```python
from build123d import *
from build123d import SkipClean  # not in build123d's __all__

# Parameters (mm, degrees)
F0_W             = 57.5
F0_H             = 50
F1_DEPTH         = 107.5
F2_W             = 55.8
F2_H             = 19
F3_DEPTH         = 42
F4_W             = 0.3
F4_H             = 19
F5_DEPTH         = 48.3
F6_T1_DEPTH      = 65.5
F6_T3_DEPTH      = 67.5
F6_T5_DEPTH      = 225
F6_T7_DEPTH      = 11.7
F6_T9_DEPTH      = 11.7
F6_T11_DEPTH     = 204
F8_W             = 87
F8_H             = 15.3
F9_DEPTH         = 14
F10_W            = 8.2
F10_H            = 14
F11_DEPTH        = 7.4
F12_R            = 2
F13_R            = 2.5
F14_DEPTH        = 4
F15_R            = 1
F19_D            = 3.3
F19_DEPTH        = 5
F19_TIP          = 0.9914200214
F19_ON_F18_D     = 3.3
F19_ON_F18_DEPTH = 5
F19_ON_F18_TIP   = 0.9914200214
F19_ON_F17_D     = 3.3
F19_ON_F17_DEPTH = 5
F19_ON_F17_TIP   = 0.9914200214
F20_W            = 264
F20_H            = 50
F20_R            = 1.5
F21_DEPTH        = 6
F22_W            = 122
F22_H            = 91
F22_R            = 2.25
F23_DEPTH        = 2.4
F24_W            = 91
F24_H            = 52.9
F24_R            = 1.75
F25_DEPTH        = 2.4
F26_R            = 2.25
F27_DEPTH        = 25
F28_W            = 91
F28_H            = 52.9
F29_DEPTH        = 3
F30_R            = 1.75
F31_DEPTH        = 25
F32_W            = 127.4
F32_H            = 91
F33_DEPTH        = 2.4
F34_W            = 127.4
F34_H            = 55.3
F34_R            = 6.5
F35_DEPTH        = 2.4
F36_W            = 21.5
F36_H            = 28.5
F37_DEPTH        = 25
F38_W            = 20
F38_H            = 100
F39_DEPTH        = 60
F43_W            = 2.4
F43_H            = 50.5
F44_DEPTH        = 45


# Not quite as in the source:
# - a fillet or chamfer that OpenCascade refuses, or shapes differently, is made with other operations: its cross-section is extruded or revolved along the edge and cut away or added


with BuildPart() as f1:
    # F0 (on Front) → F1 (new body, symmetric)
    with BuildSketch(Plane.XZ):
        with Locations((-28.75, 0)):
            Rectangle(F0_W, F0_H)
    extrude(amount=F1_DEPTH, both=True)

    # F2 (on face) → F3 (cut)
    with BuildSketch(Plane.XY.offset(25)):
        with Locations((-27.9, -98)):
            Rectangle(F2_W, F2_H)
    extrude(amount=-F3_DEPTH, mode=Mode.SUBTRACT)

    # F4 (on face) → F5 (cut)
    with BuildSketch(Plane.XY.offset(25)):
        Polygon((-55.8, 107.5), (-55.8, -88.5), (-55.5, -88.5), (-55.5, 105.5), (0, 105.5), (0, 105.8), (-55.5, 105.8), (-55.5, 107.5), align=None)
        with Locations((-55.65, -98)):
            Rectangle(F4_W, F4_H)
    extrude(amount=-F5_DEPTH, mode=Mode.SUBTRACT)

    # F6: fillet of radius 2 on 9 edges, made by hand

    # F6_s2 → F6_t1 (cut)
    with BuildSketch(Plane.YZ.offset(-60.5)):
        with BuildLine():
            ThreePointArc((-86.5, 25), (-87.9142135624, 24.4142135624), (-88.5, 23))
            Line((-88.5, 23), (-88.5, 25))
            Line((-88.5, 25), (-86.5, 25))
        make_face()
        with BuildLine():
            ThreePointArc((103.5, 25), (104.9142135624, 24.4142135624), (105.5, 23))
            Line((105.5, 23), (105.5, 25))
            Line((105.5, 25), (103.5, 25))
        make_face()
    extrude(amount=F6_T1_DEPTH, mode=Mode.SUBTRACT)

    # F6_s4 → F6_t3 (cut)
    with BuildSketch(Plane.YZ.offset(-62.5)):
        with BuildLine():
            ThreePointArc((-105.5, -25), (-106.9142135624, -24.4142135624), (-107.5, -23))
            Line((-107.5, -23), (-107.5, -25))
            Line((-107.5, -25), (-105.5, -25))
        make_face()
        with BuildLine():
            ThreePointArc((105.5, -25), (106.9142135624, -24.4142135624), (107.5, -23))
            Line((107.5, -23), (107.5, -25))
            Line((107.5, -25), (105.5, -25))
        make_face()
    extrude(amount=F6_T3_DEPTH, mode=Mode.SUBTRACT)

    # F6_s6 → F6_t5 (cut)
    with BuildSketch(Plane.XZ.offset(-112.5)):
        with BuildLine():
            ThreePointArc((-55.5, -25), (-56.9142135624, -24.4142135624), (-57.5, -23))
            Line((-57.5, -23), (-57.5, -25))
            Line((-57.5, -25), (-55.5, -25))
        make_face()
    extrude(amount=F6_T5_DEPTH, mode=Mode.SUBTRACT)

    # F6_s8 → F6_t7 (cut)
    with BuildSketch(Plane.YZ.offset(-62.5)):
        with BuildLine():
            ThreePointArc((-105.5, 25), (-106.9142135624, 24.4142135624), (-107.5, 23))
            Line((-107.5, 23), (-107.5, 25))
            Line((-107.5, 25), (-105.5, 25))
        make_face()
        with BuildLine():
            ThreePointArc((105.5, 25), (106.9142135624, 24.4142135624), (107.5, 23))
            Line((107.5, 23), (107.5, 25))
            Line((107.5, 25), (105.5, 25))
        make_face()
    extrude(amount=F6_T7_DEPTH, mode=Mode.SUBTRACT)

    # F6_s10 → F6_t9 (cut)
    with BuildSketch(Plane.XZ.offset(-112.5)):
        with BuildLine():
            ThreePointArc((-55.5, 23), (-54.9142135624, 24.4142135624), (-53.5, 25))
            Line((-53.5, 25), (-55.5, 25))
            Line((-55.5, 25), (-55.5, 23))
        make_face()
    extrude(amount=F6_T9_DEPTH, mode=Mode.SUBTRACT)

    # F6_s12 → F6_t11 (cut)
    with BuildSketch(Plane.XZ.offset(-110.5)):
        with BuildLine():
            ThreePointArc((-53.5, 25), (-54.9142135624, 24.4142135624), (-55.5, 23))
            Line((-55.5, 23), (-55.5, 25))
            Line((-55.5, 25), (-53.5, 25))
        make_face()
    with SkipClean():  # cleaning this boolean's faces spoils the solid; the shape is the same uncleaned
        extrude(amount=F6_T11_DEPTH, mode=Mode.SUBTRACT)

    # F7: F1 across plane


with BuildPart() as f1_1:
    add(f1.part, clean=False)
    add(f1.part.mirror(Plane.YZ), clean=False)

    # F19
    with Locations(Plane(origin=(-57.5, 0, 0), x_dir=(0, -1, 0), z_dir=(-1, 0, 0))):
        with Locations((-75, -13), (75, -13)):
            Hole(F19_D / 2, depth=F19_DEPTH)
            with Locations((0, 0, -(F19_DEPTH + F19_TIP / 2))):  # 118° drill point
                Cone(0, F19_D / 2, F19_TIP, mode=Mode.SUBTRACT)

    # F19 on F18
    with Locations(Plane(origin=(0, 0, -25), x_dir=(1, 0, 0), z_dir=(0, 0, -1))):
        with Locations((-25, -75), (-25, 75), (25, -75), (25, 75)):
            Hole(F19_ON_F18_D / 2, depth=F19_ON_F18_DEPTH)
            with Locations((0, 0, -(F19_ON_F18_DEPTH + F19_ON_F18_TIP / 2))):  # 118° drill point
                Cone(0, F19_ON_F18_D / 2, F19_ON_F18_TIP, mode=Mode.SUBTRACT)

    # F19 on F17
    with Locations(Plane.YZ.offset(57.5)):
        with Locations((-75, -13), (-75, 12), (75, 12), (75, -13)):
            Hole(F19_ON_F17_D / 2, depth=F19_ON_F17_DEPTH)
            with Locations((0, 0, -(F19_ON_F17_DEPTH + F19_ON_F17_TIP / 2))):  # 118° drill point
                Cone(0, F19_ON_F17_D / 2, F19_ON_F17_TIP, mode=Mode.SUBTRACT)


with BuildPart() as f9:
    # F8 (on face) → F9 (new body)
    with BuildSketch(Plane.XY.offset(-17)):
        with Locations((9.3, -96.15)):
            Rectangle(F8_W, F8_H)
    extrude(amount=F9_DEPTH)

    # F10 (on face) → F11 (cut)
    with BuildSketch(Plane.XY.offset(-3)):
        with Locations((-28.7, -96.8)):
            Rectangle(F10_W, F10_H)
        with Locations((-19.2, -96.8)):
            Rectangle(F10_W, F10_H)
        with Locations((-9.7, -96.8)):
            Rectangle(F10_W, F10_H)
        with Locations((-0.2, -96.8)):
            Rectangle(F10_W, F10_H)
        with Locations((9.3, -96.8)):
            Rectangle(F10_W, F10_H)
        with Locations((18.8, -96.8)):
            Rectangle(F10_W, F10_H)
        with Locations((28.3, -96.8)):
            Rectangle(F10_W, F10_H)
        with Locations((37.8, -96.8)):
            Rectangle(F10_W, F10_H)
        with Locations((47.3, -96.8)):
            Rectangle(F10_W, F10_H)
    extrude(amount=-F11_DEPTH, mode=Mode.SUBTRACT)

    # F12
    f12_edges = [f9.edges().sort_by_distance(p)[0] for p in [
        (-33.5, -103.8, -3),
        (-23.95, -103.8, -3),
        (-14.45, -103.8, -3),
        (-4.95, -103.8, -3),
        (4.55, -103.8, -3),
        (14.05, -103.8, -3),
        (23.55, -103.8, -3),
        (33.05, -103.8, -3),
        (42.55, -103.8, -3),
        (52.1, -103.8, -3),
    ]]
    fillet(f12_edges, radius=F12_R)

    # F13 (on face) → F14 (join)
    with BuildSketch(Plane.XY.offset(-10.4)):
        with Locations((-28.7, -96.8)):
            Circle(F13_R)
        with Locations((-19.2, -96.8)):
            Circle(F13_R)
        with Locations((-9.7, -96.8)):
            Circle(F13_R)
        with Locations((-0.2, -96.8)):
            Circle(F13_R)
        with Locations((9.3, -96.8)):
            Circle(F13_R)
        with Locations((18.8, -96.8)):
            Circle(F13_R)
        with Locations((28.3, -96.8)):
            Circle(F13_R)
        with Locations((37.8, -96.8)):
            Circle(F13_R)
        with Locations((47.3, -96.8)):
            Circle(F13_R)
    extrude(amount=F14_DEPTH)

    # F15
    f15_edges = [f9.edges().sort_by_distance(p)[0] for p in [
        (-31.2, -96.8, -6.4),
        (-21.7, -96.8, -6.4),
        (-12.2, -96.8, -6.4),
        (-2.7, -96.8, -6.4),
        (6.8, -96.8, -6.4),
        (16.3, -96.8, -6.4),
        (25.8, -96.8, -6.4),
        (35.3, -96.8, -6.4),
        (44.8, -96.8, -6.4),
    ]]
    fillet(f15_edges, radius=F15_R)


with BuildPart() as f21:
    # F20 (on face) → F21 (new body)
    with BuildSketch(Plane.YZ.offset(57.5)):
        with Locations((-24.5, 0)):
            Rectangle(F20_W, F20_H)
        with Locations((-75, -13)):
            Circle(F20_R, mode=Mode.SUBTRACT)
        with Locations((75, -13)):
            Circle(F20_R, mode=Mode.SUBTRACT)
        with Locations((-75, 12)):
            Circle(F20_R, mode=Mode.SUBTRACT)
        with Locations((75, 12)):
            Circle(F20_R, mode=Mode.SUBTRACT)
    extrude(amount=F21_DEPTH)


with BuildPart() as f23:
    # F22 (on face) → F23 (new body)
    with BuildSketch(Plane(origin=(0, 0, -25), x_dir=(1, 0, 0), z_dir=(0, 0, -1))):
        with Locations((3, 111.9773719933)):
            Rectangle(F22_W, F22_H)
        with Locations((-25, 75)):
            Circle(F22_R, mode=Mode.SUBTRACT)
        with Locations((25, 75)):
            Circle(F22_R, mode=Mode.SUBTRACT)
    extrude(amount=F23_DEPTH)

    # F24 (on face) → F25 (join)
    with BuildSketch(Plane(origin=(-58, 0, 0), x_dir=(0, -1, 0), z_dir=(-1, 0, 0))):
        with Locations((111.9773719933, -0.95)):
            Rectangle(F24_W, F24_H)
        with Locations((137.4773719933, -19.75)):
            Circle(F24_R, mode=Mode.SUBTRACT)
        with BuildLine():
            Line((127.4773719933, 9.25), (132.4773719933, 14.25))
            Line((132.4773719933, 14.25), (142.4773719933, 14.25))
            ThreePointArc((142.4773719933, 14.25), (146.0129058993, 12.7855339059), (147.4773719933, 9.25))
            Line((147.4773719933, 9.25), (147.4773719933, -8.75))
            ThreePointArc((147.4773719933, -8.75), (146.0129058993, -12.2855339059), (142.4773719933, -13.75))
            Line((142.4773719933, -13.75), (132.4773719933, -13.75))
            Line((132.4773719933, -13.75), (127.4773719933, -8.75))
            Line((127.4773719933, -8.75), (127.4773719933, 9.25))
        make_face(mode=Mode.SUBTRACT)
        with Locations((137.4773719933, 20.25)):
            Circle(F24_R, mode=Mode.SUBTRACT)
    extrude(amount=F25_DEPTH)

    # F26 (on face) → F27 (cut)
    with BuildSketch(Plane(origin=(-57.5, 0, 0), x_dir=(0, -1, 0), z_dir=(-1, 0, 0))):
        with Locations((75, -13)):
            Circle(F26_R)
    extrude(amount=F27_DEPTH, mode=Mode.SUBTRACT)

    # F28 (on face) → F29 (join)
    with BuildSketch(Plane.YZ.offset(64)):
        with Locations((-111.9773719933, -0.95)):
            Rectangle(F28_W, F28_H)
    extrude(amount=F29_DEPTH)

    # F30 (on face) → F31 (cut)
    with BuildSketch(Plane.YZ.offset(63.5)):
        with Locations((-75, 12)):
            Circle(F30_R)
        with Locations((-75, -13)):
            Circle(F30_R)
    extrude(amount=F31_DEPTH, mode=Mode.SUBTRACT)

    # F32 (on face) → F33 (join)
    with BuildSketch(Plane.XY.offset(25.5)):
        with Locations((3.3, -111.9773719933)):
            Rectangle(F32_W, F32_H)
    extrude(amount=F33_DEPTH)

    # F34 (on face) → F35 (join)
    with BuildSketch(Plane.XZ.offset(157.4773719933)):
        with Locations((3.3, 0.25)):
            Rectangle(F34_W, F34_H)
        with Locations((-8, 5.5)):
            Circle(F34_R, mode=Mode.SUBTRACT)
    extrude(amount=F35_DEPTH)

    # F36 (on face) → F37 (cut)
    with BuildSketch(Plane(origin=(0, 0, -27.4), x_dir=(1, 0, 0), z_dir=(0, 0, -1))):
        with Locations((16.25, 133.2273719933)):
            Rectangle(F36_W, F36_H)
    extrude(amount=-F37_DEPTH, mode=Mode.SUBTRACT)


with BuildPart() as f39_tool:
    # F38 (on face) → F39 (new body)
    with BuildSketch(Plane.XY.offset(27.9)):
        with Locations((57, -109.8773719933)):
            Rectangle(F38_W, F38_H)
    extrude(amount=-F39_DEPTH)


with BuildPart() as f1_2:
    add(f1_1.part, clean=False)

    # F39: cut by f39_tool
    add(f39_tool.part, mode=Mode.SUBTRACT)


with BuildPart() as f9_1:
    add(f9.part, clean=False)

    # F39: cut by f39_tool
    add(f39_tool.part, mode=Mode.SUBTRACT)


with BuildPart() as f21_1:
    add(f21.part, clean=False)

    # F39: cut by f39_tool
    add(f39_tool.part, mode=Mode.SUBTRACT)


with BuildPart() as f23_1:
    add(f23.part, clean=False)

    # F39: cut by f39_tool
    add(f39_tool.part, mode=Mode.SUBTRACT)

    # F43 (on face) → F44 (join)
    with BuildSketch(Plane(origin=(0, -157.4773719933, 0), x_dir=(-1, 0, 0), z_dir=(0, 1, 0))):
        with Locations((-45.8, 0.25)):
            Rectangle(F43_W, F43_H)
    extrude(amount=F44_DEPTH)


solid = f23_1.part
```
The model under review builds one solid part; all positions refer to its coordinate system, in mm. A direction names the side the tool comes from. Round coordinates to 2 decimals unless told otherwise and drop trailing zeros. Loops run counter-clockwise (first coordinate to the right, second up) from the corner with the lowest first, then second, coordinate; pieces in that order, holes last. Notation, with made-up numbers: M 74,51 L 90,51 A17 ccw 90,70 Z; hole C 46,41.5 d2. An arc over 180 degrees is marked long. Answer as a JSON object with one key per item and string values.
(1) Take a section at A-A on x = 25. Give the boundary of the cut face in (y, z), and give its area (3 significant figures).
Resolved:
{"outline": "M -159.88,-27.4 L -147.48,-27.4 L -147.48,-25 L -157.48,-25 L -157.48,25.5 L -66.48,25.5 L -66.48,27.9 L -159.88,27.9 Z; M -118.98,-27.4 L -77.25,-27.4 L -77.25,-25 L -118.98,-25 Z; M -72.75,-27.4 L -66.48,-27.4 L -66.48,-25 L -72.75,-25 Z", "area": "490 mm²"}
(2) Take a section at B-B on z = 5.5. Give the boundary of the cut face in (x, y).
Resolved:
{"outline": "M -60.4,-159.88 L -14.5,-159.88 L -14.5,-157.48 L -58,-157.48 L -58,-147.48 L -60.4,-147.48 Z; M -60.4,-127.48 L -58,-127.48 L -58,-66.48 L -60.4,-66.48 Z; M -1.5,-159.88 L 47,-159.88 L 47,-112.48 L 44.6,-112.48 L 44.6,-157.48 L -1.5,-157.48 Z"}
(3) Clearance check with flat-ended pins moving along their axes: P1, Ø1.9, axis at x = 45.5, z = 7, coming from the +Y side; P2, Ø6, axis at x = -5.5, z = 2.5, coming from the +Y side; P3, Ø4, axis at x = 14.5, y = -129, coming from the -Z side. State where each tip first meets the part, or that it passes through.
Resolved:
{"P1": "y = -112.48", "P2": "y = -157.48", "P3": "z = 25.5"}
(4) Take a section at C-C on x = -25. Give the boundary of the cut face in (y, z), and give its area (3 significant figures).
Resolved:
{"outline": "M -159.88,-27.4 L -77.25,-27.4 L -77.25,-25 L -157.48,-25 L -157.48,25.5 L -66.48,25.5 L -66.48,27.9 L -159.88,27.9 Z; M -72.75,-27.4 L -66.48,-27.4 L -66.48,-25 L -72.75,-25 Z", "area": "559 mm²"}
(5) Draft analysis for pull direction X (two halves, no side actions). For faces 4 (the flat face through (47, -135, 0)), 5 (the cylindrical face through (24.512, -72.804, -26.183)), 6 (the flat face through (-59.183, -129.942, 11.715)), state which applies: released by +X, released by -X, zero draft, split by the parting line, or undercut.
Resolved:
{"face 4": "released by +X", "face 5": "undercut", "face 6": "zero draft"}
(6) Take a section at D-D on y = -75. Give the boundary of the cut face in (x, z), and give its area (3 significant figures).
Resolved:
{"outline": "M -60.4,-27.4 L -27.25,-27.4 L -27.25,-25 L -58,-25 L -58,-15.25 L -60.4,-15.25 Z; M -60.4,-10.75 L -58,-10.75 L -58,25.5 L 47,25.5 L 47,27.9 L -60.4,27.9 Z; M -22.75,-27.4 L 22.75,-27.4 L 22.75,-25 L -22.75,-25 Z; M 27.25,-27.4 L 47,-27.4 L 47,-25 L 27.25,-25 Z", "area": "604 mm²"}
(7) Tool access review of faces 1 (the flat face through (-58, -111, 1)), 2 (the flat face through (27, -133, -26)), 3 (the cylindrical face through (-59.183, -139.147, -19.224)): name each direction out of +Z, -Z, +X, -X, +Y, -Y from which nothing blocks a thin tool from reaching the whole face with its end or side.
Resolved:
{"face 1": "+Y", "face 2": "-Z", "face 3": "-X"}
(8) To check wall thickness, follow line 1 along Y through (x, z) = (-25, -25.9); line 2 along Z through (x, y) = (20.5, -97.5); line 3 along X through (y, z) = (-153, 24). State the ranges of each line that lie inside material, in increasing order.
Resolved:
{"line 1": "-159.88 to -77.25, -72.75 to -66.48", "line 2": "-27.4 to -25, 25.5 to 27.9", "line 3": "-60.4 to -58, 44.6 to 47"}
